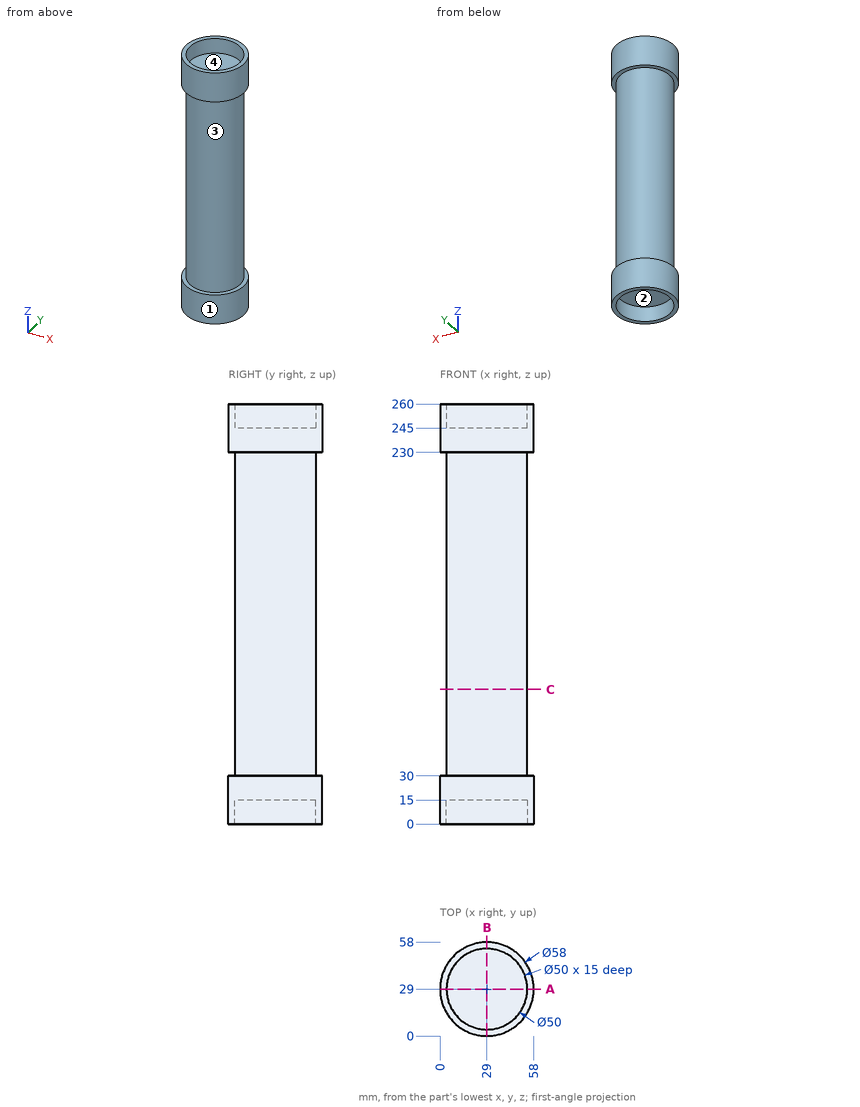
Input: dimensioned drawing with shaded views. Units: mm. Origin: part minimum x, y, z. A direction names the side the tool comes from. Coordinates: 2 decimals unless noted, no trailing zeros. Loops run counter-clockwise (first coordinate to the right, second up) from the corner with the lowest first, then second, coordinate; pieces in that order, holes last. Notation, with made-up numbers: M 86,56.25 L 145,56.25 A18 cw 145,90.25 Z; hole C 62.25,-29.5 d3. An arc over 180 degrees is marked long. One line per item, written item: value.
(1) Pull-direction query (X, two-part tool) for the marked faces 3 and 4; classes: +X half, -X half, draft (parallel to the pull), parting line (faces both ways), or undercut.
Filled in:
face 3: parting line
face 4: undercut
(2) Section C-C (z = 83.5). Output: boundary loops of the cut face in (x, y), and give its area (3 significant figures).
Filled in:
outline: C 29,29 d50
area: 1,960 mm^2
(3) Line query: line 1 along Z through (x, y) = (15.5, 6.5); line 2 along Y through (x, z) = (29, 9.75); line 3 along Z through (x, y) = (31, 46.5). Output: solid intervals per line, ascending. Write a range as from..to.
Filled in:
line 1: 0..30, 230..260
line 2: 0..4, 54..58
line 3: 15..245
(4) Section A-A (y = 29). Output: boundary loops of the cut face in (x, z), and give its area (3 significant figures).
Filled in:
outline: M 0,0 L 4,0 L 4,15 L 54,15 L 54,0 L 58,0 L 58,30 L 54,30 L 54,230 L 58,230 L 58,260 L 54,260 L 54,245 L 4,245 L 4,260 L 0,260 L 0,230 L 4,230 L 4,30 L 0,30 Z
area: 12,000 mm^2
(5) Reachability of the marked faces 1 and 2 from +Z, -Z, +X, -X, +Y, -Y: full face, straight path, thin tool, end or side. Return the list, or none.
Filled in:
face 1: +Z, -Z
face 2: -Z
(6) Pin query (flat end, axial travel): pin 1 (4 mm diameter, centred on y = 30.5, z = 227.5, fed in from -X); pin 2 (25 mm diameter, centred on x = 30.5, y = 37.5, fed in from +Z); pin 3 (1 mm diameter, centred on x = 38, y = 45.5, fed in from -Z). Return the tip coordinate at first contact, or that it passes through.
Filled in:
pin 1: x = 4
pin 2: z = 245
pin 3: z = 15
